Geometry: see drawing. Coordinates: mm, zero at the bounding-box minimum. A direction names the side the tool comes from. Give positions to 0.01 mm unless a question says otherwise; leave off trailing zeros. Order: outer loops, then holes, each group sorted by start corner. A loop starts at its lowest first (then second) coordinate and runs counter-clockwise, first axis right, second up. Notation, with made-up numbers: (26, -31) - (83, -31) arc R36 ccw to (83, 3) - close; hole circle Ø2 at (-7.75, -23.75). An arc over 180 degrees is marked (long way). One line per item, written item: value.
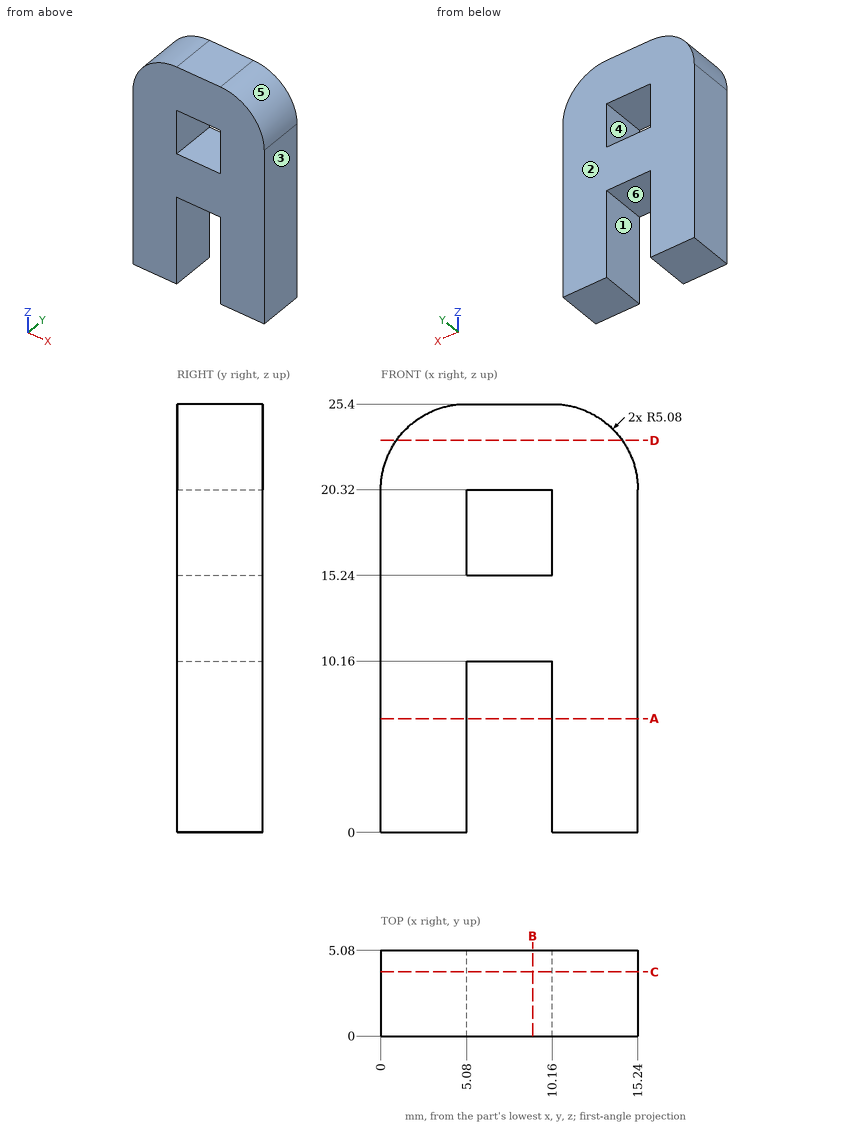
1) Section A-A, the plane z = 6.75. Return loops of the section in (x, y), then the cut area to 3 significant figures.
Answers below:
outline: (0, 0) - (5.08, 0) - (5.08, 5.08) - (0, 5.08) - close; (10.16, 0) - (15.24, 0) - (15.24, 5.08) - (10.16, 5.08) - close
area: 51.6 mm^2
2) Section B-B, the plane x = 9. Return loops of the section in (y, z), then the cut area to 3 significant figures.
Answers below:
outline: (0, 10.16) - (5.08, 10.16) - (5.08, 15.24) - (0, 15.24) - close; (0, 20.32) - (5.08, 20.32) - (5.08, 25.4) - (0, 25.4) - close
area: 51.6 mm^2
3) Material intervals for line 1 along Z through (x, y) = (7.25, 1.45); line 2 along X through (y, z) = (0.5, 8.5); line 3 along Z through (x, y) = (1, 2.2), sorted ascending.
Answers below:
line 1: 10.16 to 15.24, 20.32 to 25.4
line 2: 0 to 5.08, 10.16 to 15.24
line 3: 0 to 23.35
4) Section C-C, the plane y = 3.8. Return loops of the section in (x, z), then the cut area to 3 significant figures.
Answers below:
outline: (0, 0) - (5.08, 0) - (5.08, 10.16) - (10.16, 10.16) - (10.16, 0) - (15.24, 0) - (15.24, 20.32) arc R5.08 ccw to (10.16, 25.4) - (5.08, 25.4) arc R5.08 ccw to (0, 20.32) - close; hole (5.08, 15.24) - (10.16, 15.24) - (10.16, 20.32) - (5.08, 20.32) - close
area: 299 mm^2
5) Section D-D, the plane z = 23.25. Return loops of the section in (x, y), then the cut area to 3 significant figures.
Answers below:
outline: (0.93, 0) - (14.31, 0) - (14.31, 5.08) - (0.93, 5.08) - close
area: 68.0 mm^2
6) Mould query, pull axis X, two halves, no side actions, for the marked faces 1, 2 and 3. Classes: released by +X, released by -X, zero draft, split by the parting line, or undercut.
Answers below:
face 1: undercut
face 2: zero draft
face 3: released by +X
7) Set-up query: the marked faces 4, 5 and 6. Return all of +Z, -Z, +X, -X, +Y, -Y with unobstructed straight access to the full face (end or side cutting, diameter ignored); none if empty.
Answers below:
face 4: +Y, -Y
face 5: +Z, +X, +Y, -Y
face 6: -Z, +Y, -Y
